The listing builds one solid part. Answer for the finished solid, in the listing's coordinates (mm). Face numbers are marked on the shaded views. A direction names the side the tool comes from. Give positions to 0.01 mm unless a question says otherwise; leave off trailing zeros. Order: outer loops, then holes, each group sorted by start corner. A loop starts at its lowest first (then second) coordinate and runs counter-clockwise, first axis right, second up. Notation, with made-up numbers: (1, -12) -> (19, -12) arc R11 ccw to (19, 6) -> close; hole circle Ø9 at (-25, 83). An arc over 180 degrees is marked (long way). One line per question, with ' | ' between items. Start each with the question number.
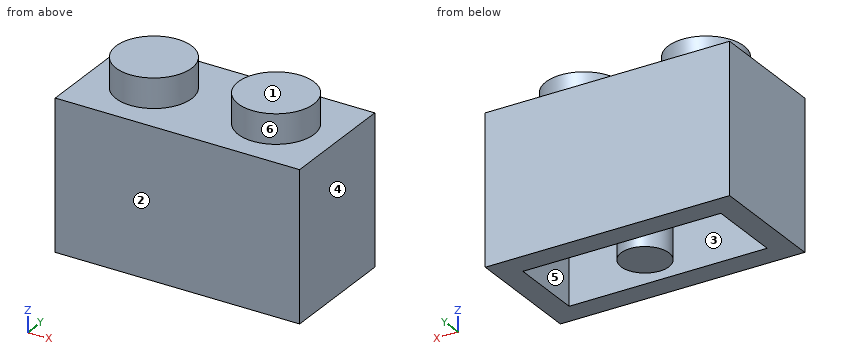
```python
from build123d import *

# Parameters (mm, degrees)
F0_W     = 15.8
F0_H     = 9.6
F1_DEPTH = 7.8
F2_R     = 2.45
F3_DEPTH = 1.9
F4_W     = 12.8
F4_H     = 4.8
F4_R     = 1.55
F5_DEPTH = 8.3


with BuildPart() as f1:
    # F0 (on Front) → F1 (new body)
    with BuildSketch(Plane.XZ):
        with Locations((-56.280687, -17.648849)):
            Rectangle(F0_W, F0_H)
    extrude(amount=F1_DEPTH)

    # F2 (on face) → F3 (join)
    with BuildSketch(Plane.XY.offset(-12.848849)):
        with Locations((-60.230687, -3.9)):
            Circle(F2_R)
        with Locations((-52.330687, -3.9)):
            Circle(F2_R)
    extrude(amount=F3_DEPTH)

    # F4 (on face) → F5 (cut)
    with BuildSketch(Plane(origin=(0, 0, -22.448849), x_dir=(1, 0, 0), z_dir=(0, 0, -1))):
        with Locations((-56.280687, 3.9)):
            Rectangle(F4_W, F4_H)
        with Locations((-56.280687, 3.9)):
            Circle(F4_R, mode=Mode.SUBTRACT)
    extrude(amount=-F5_DEPTH, mode=Mode.SUBTRACT)


solid = f1.part
```
(1) The part is cut by section D-D on x = -57.25. Determine the outline of the cut face in (y, z), plus the area to 3 significant figures.
(2) Determine the mould class of the marked faces 1, 2 and 3 for opening direction Y: pulls with the +Y half, pulls with the -Y half, needs draft (parallel to the pull), parting line crosses it, or undercut.
(3) The part is cut by section A-A on z = -20.5. Determine the outline of the cut face in (x, y).
(4) The part is cut by section C-C on x = -53.5. Determine the outline of the cut face in (y, z), plus the area to 3 significant figures.
(5) Given P1, Ø3, axis at x = -60, z = -19.5, coming from the +Y side, flat-ended and moving along its own axis, determine where the tip first touches the part or whether it passes through.
(6) Consider line 1 (X direction, y = -4, z = -19.75); line 2 (Y direction, x = -58.5, z = -16); line 3 (X direction, y = -3.25, z = -19.5). Determine where each line is inside the solid, lowest interval first.
(7) The part is cut by section B-B on y = -3.9. Determine the outline of the cut face in (x, z).
(8) For the marked faces 4, 5 and 6, determine the directions among +Z, -Z, +X, -X, +Y, -Y from which every point of the face is accessible in a straight line to the end or side of a thin tool.
Result sheet:
1) outline: (-7.8, -22.45) -> (-6.3, -22.45) -> (-6.3, -14.15) -> (-5.11, -14.15) -> (-5.11, -22.45) -> (-2.69, -22.45) -> (-2.69, -14.15) -> (-1.5, -14.15) -> (-1.5, -22.45) -> (0, -22.45) -> (0, -12.85) -> (-7.8, -12.85) -> close | area: 55.1 mm^2
2) face 1: needs draft | face 2: pulls with the -Y half | face 3: undercut
3) outline: (-64.18, -7.8) -> (-48.38, -7.8) -> (-48.38, 0) -> (-64.18, 0) -> close; circle Ø3.1 at (-56.28, -3.9); hole (-62.68, -6.3) -> (-49.88, -6.3) -> (-49.88, -1.5) -> (-62.68, -1.5) -> close
4) outline: (-7.8, -22.45) -> (-6.3, -22.45) -> (-6.3, -14.15) -> (-1.5, -14.15) -> (-1.5, -22.45) -> (0, -22.45) -> (0, -12.85) -> (-1.75, -12.85) -> (-1.75, -10.95) -> (-6.05, -10.95) -> (-6.05, -12.85) -> (-7.8, -12.85) -> close | area: 43.2 mm^2
5) P1: stops at y = 0
6) line 1: x = -64.18 to -62.68, -57.83 to -54.73, -49.88 to -48.38 | line 2: y = -7.8 to -6.3, -1.5 to 0 | line 3: x = -64.18 to -62.68, -57.69 to -54.87, -49.88 to -48.38
7) outline: (-64.18, -22.45) -> (-62.68, -22.45) -> (-62.68, -14.15) -> (-57.83, -14.15) -> (-57.83, -22.45) -> (-54.73, -22.45) -> (-54.73, -14.15) -> (-49.88, -14.15) -> (-49.88, -22.45) -> (-48.38, -22.45) -> (-48.38, -12.85) -> (-49.88, -12.85) -> (-49.88, -10.95) -> (-54.78, -10.95) -> (-54.78, -12.85) -> (-57.78, -12.85) -> (-57.78, -10.95) -> (-62.68, -10.95) -> (-62.68, -12.85) -> (-64.18, -12.85) -> close
8) face 4: +Z, -Z, +X, +Y, -Y | face 5: -Z | face 6: +Z
